Autodesk Inventor part; units mm, degrees
ref_plane "YZ Plane" through (0, 0, 0) normal (1, 0, 0) x (0, 1, 0)
ref_plane "XZ Plane" through (0, 0, 0) normal (0, 1, 0) x (-1, 0, 0)
ref_plane "XY Plane" through (0, 0, 0) normal (0, 0, 1) x (1, 0, 0)
sketch "Sketch1" plane through (0, 0, 0) normal (0, 0, 1) x (1, 0, 0)
  line L0 (0, 0) -> (63.5, 0)
  line L1 (63.5, 0) -> (63.5, 50.8)
  line L2 (63.5, 50.8) -> (0, 50.8)
  line L3 (0, 50.8) -> (0, 0)
  dimension "d0" = 50.8
  dimension "d1" = 63.5
extrude "Extrusion1" add sketch "Sketch1" along normal blind 1.27
sketch "Sketch2" plane through (0, 0, 1.27) normal (0, 0, 1) x (1, 0, 0)
  line L0 (63.5, 0) -> (63.5, 50.8)
  line L1 (0, 0) -> (63.5, 0)
  line L2 (63.5, 0) -> (63.5, 2.54)
  line L3 (63.5, 2.54) -> (0, 2.54)
  line L4 (0, 2.54) -> (0, 0)
  dimension "d4" = 2.54
extrude "Extrusion2" add sketch "Sketch2" along normal blind 6.35
sketch "Sketch3" plane through (0, 0, 1.27) normal (0, 0, 1) x (1, 0, 0)
  line L0 (63.5, 50.8) -> (0, 50.8)
  line L1 (63.5, 2.54) -> (63.5, 50.8)
  point P0 (0, 0)
  point P1 (31.75, 33.02)
  dimension "d7" = 17.78
  dimension "d8" = 31.75
hole "Hole1" at (31.75, 33.02, 1.27) direction (0, 0, -1) diameter 3.175 depth 25.4 tip angle 118
sketch "Sketch4" plane through (0, 0, 1.27) normal (0, 0, 1) x (1, 0, 0)
  line L0 (0, 50.8) -> (0, 2.54)
  line L1 (63.5, 2.54) -> (63.5, 50.8)
  line L2 (63.5, 50.8) -> (0, 50.8)
  point P0 (0, 0)
  point P1 (5.08, 45.72)
  point P2 (58.42, 45.72)
  dimension "d16" = 5.08
  dimension "d17" = 5.08
  dimension "d18" = 5.08
  dimension "d19" = 5.08
hole "Hole2" at (5.08, 45.72, 1.27) at (58.42, 45.72, 1.27) direction (0, 0, -1) diameter 3.1852 depth 25.4 tip angle 118
sketch "Sketch5" plane through (0, 2.54, 1.27) normal (0, 1, 0) x (1, 0, 0)
  line L0 (63.5, -6.35) -> (0, -6.35)
  line L1 (0, 0) -> (0, -6.35)
  line L2 (63.5, 0) -> (63.5, -6.35)
  point P0 (0, 1.27)
  point P1 (5.08, -3.175)
  point P2 (58.42, -3.175)
  dimension "d27" = 3.175
  dimension "d28" = 5.08
  dimension "d29" = 3.175
  dimension "d30" = 5.08
hole "Hole3" at (5.08, 2.54, 4.445) at (58.42, 2.54, 4.445) direction (0, -1, 0) diameter 3.1852 depth 25.4 tip angle 118
sketch "Sketch6" plane through (0, 0, 1.27) normal (0, 0, 1) x (1, 0, 0)
  circle A0 centre (31.75, 33.02) radius 1.5875 construction
  circle A1 centre (31.75, 33.02) radius 3.81 construction
  circle A2 centre (27.8616, 26.4668) radius 3.81 construction
  line L0 (63.5, 2.54) -> (0, 2.54) construction
  circle A3 centre (27.8616, 26.4668) radius 1.5875
  line L1 (0, 0) -> (63.5, 0)
  dimension "d39" = 7.62
  dimension "d40" = 7.62
  dimension "d42" = 3.175
  dimension "d47" = 26.4668
extrude "Extrusion3" cut sketch "Sketch6" against normal blind 25.4
properties part number "000110-1"
Here's how the part is built. I have some questions about the finished solid (model axes, mm). A direction names the side the tool comes from. Give positions to 0.01 mm unless a question says otherwise; leave off trailing zeros. Order: outer loops, then holes, each group sorted by start corner. A loop starts at its lowest first (then second) coordinate and runs counter-clockwise, first axis right, second up. Notation, with made-up numbers: (-28, 71.25) -> (-9, 71.25) arc R22 ccw to (-9, 106.25) -> close; hole circle Ø7 at (1.25, 52). An arc over 180 degrees is marked (long way). Use CSV: the item, a comma, the result in double quotes. Start each with the question number.
Item 1: Suppose I cut it at C-C (x = 31.75). List the corners of the cut face in (y, z) for me, and give its area (3 significant figures).
Item 2: Suppose I cut it at D-D (y = 33.02). List the corners of the cut face in (x, z) for me, and give its area (3 significant figures).
Item 3: On a 3-axis mill with a long thin cutter (end or side, diameter ignored), from which of +Z, -Z, +X, -X, +Y, -Y can I reach the whole of each face in a straight line? I mean faces 5 (the flat face through (31, 1, 7.62)), 6 (the flat face through (31, 27, 1.27)). Say none if no direction works.
Item 4: Suppose I cut it at B-B (y = 45.72). List the corners of the cut face in (x, z) for me, and give its area (3 significant figures).
Item 5: If I drill on probe 1 along X at (y, z) = (45.72, 0.65); probe 2 along X at (y, z) = (33.02, 0.75); probe 3 along Z at (x, y) = (5, 1), over which ranges is the centre line in solid material (lowest first)? Write a range as [from, to].
Item 6: I'm going to push flat-ended pins straight in: P1, Ø1, axis at x = 9, y = 13, coming from the -Z side; P2, Ø3, axis at x = 30.5, z = 5, coming from the +Y side; P3, Ø5, axis at x = 5.08, y = 45.72, coming from the +Z side; P4, Ø1.9, axis at x = 58.42, y = 45.72, coming from the +Z side. Where does each tip first touch, or does it pass through?
Item 7: Thinking about a two-plate mould opening in X: for faces 1 (the cylindrical face through (30.41, 32.17, 0.63)), 2 (the flat face through (63.5, 22, 1)), 3 (the flat face through (31, 26, 0)), 4 (the cylindrical face through (27.517, 24.917, 0.644)), which applies, pulls with the +X half, pulls with the -X half, needs draft (parallel to the pull), parting line crosses it, or undercut?
Item 8: Suppose I cut it at A-A (x = 58.42). List the corners of the cut face in (y, z) for me, and give its area (3 significant figures).
Answer block:
1,outline,"(0, 0) -> (31.43, 0) -> (31.43, 1.27) -> (2.54, 1.27) -> (2.54, 7.62) -> (0, 7.62) -> close; (34.61, 0) -> (50.8, 0) -> (50.8, 1.27) -> (34.61, 1.27) -> close"
1,area,"76.6 mm^2"
2,outline,"(0, 0) -> (30.16, 0) -> (30.16, 1.27) -> (0, 1.27) -> close; (33.34, 0) -> (63.5, 0) -> (63.5, 1.27) -> (33.34, 1.27) -> close"
2,area,"76.6 mm^2"
3,face 5,"+Z, +X, -X, +Y, -Y"
3,face 6,"+Z, +X, -X, +Y"
4,outline,"(0, 0) -> (3.49, 0) -> (3.49, 1.27) -> (0, 1.27) -> close; (6.67, 0) -> (56.83, 0) -> (56.83, 1.27) -> (6.67, 1.27) -> close; (60.01, 0) -> (63.5, 0) -> (63.5, 1.27) -> (60.01, 1.27) -> close"
4,area,"72.6 mm^2"
5,probe 1,"x = [0, 3.49], [6.67, 56.83], [60.01, 63.5]"
5,probe 2,"x = [0, 30.16], [33.34, 63.5]"
5,probe 3,"z = [0, 2.85], [6.04, 7.62]"
6,P1,"stops at z = 0"
6,P2,"stops at y = 2.54"
6,P3,"stops at z = 1.27"
6,P4,"passes through"
7,face 1,"undercut"
7,face 2,"pulls with the +X half"
7,face 3,"needs draft"
7,face 4,"undercut"
8,outline,"(0, 0) -> (44.13, 0) -> (44.13, 1.27) -> (2.54, 1.27) -> (2.54, 2.85) -> (0, 2.85) -> close; (0, 6.04) -> (2.54, 6.04) -> (2.54, 7.62) -> (0, 7.62) -> close; (47.31, 0) -> (50.8, 0) -> (50.8, 1.27) -> (47.31, 1.27) -> close"
8,area,"68.5 mm^2"
